```python
from build123d import *

# Parameters (mm, degrees)
FILLET1_R           = 0.2
FILLET2_R           = 1
SKETCH2_R           = 2.5
BOSS_EXTRUDE1_DEPTH = 30
CUT_EXTRUDE1_DEPTH  = 2


with BuildPart() as part:
    # Sketch1 → Revolve1 (revolve)
    with BuildSketch(Plane.XY):
        with BuildLine():
            Line((0, 0), (4.65, 0))
            Line((4.65, 0), (4.65, 1))
            ThreePointArc((4.65, 1), (3.526943142, 2.164793721), (2, 2.7))
            Line((2, 2.7), (0, 2.7))
            Line((0, 2.7), (0, 0))
        make_face()
    revolve(axis=Axis((0, 55, 0), (0, -1, 0)))

    # Fillet1
    fillet1_edges = [part.edges().sort_by_distance(p)[0] for p in [
        (-4.65, 0, 0),
    ]]
    fillet(fillet1_edges, radius=FILLET1_R)

    # Fillet2
    fillet2_edges = [part.edges().sort_by_distance(p)[0] for p in [
        (-4.65, 1, 0),
    ]]
    fillet(fillet2_edges, radius=FILLET2_R)

    # Sketch2 → Boss-Extrude1 (add)
    with BuildSketch(Plane.XZ):
        Circle(SKETCH2_R)
    extrude(amount=BOSS_EXTRUDE1_DEPTH)

    # Sketch6 → Revolve2 (revolve)
    with BuildSketch(Plane.XY):
        Polygon((0, 0), (0, 2.7), (1.274203424, 2.7), (4.45, 0), align=None)
    revolve(axis=Axis((0, 55, 0), (0, -1, 0)))

    # Sketch7 → Cut-Extrude1 (cut)
    with BuildSketch(Plane(origin=(0, 2.7, 0), x_dir=(1, 0, 0), z_dir=(0, 1, 0))):
        Polygon((0.866025404, -1.5), (1.732050808, 0), (0.866025404, 1.5), (-0.866025404, 1.5), (-1.732050808, 0), (-0.866025404, -1.5), align=None)
    extrude(amount=-CUT_EXTRUDE1_DEPTH, mode=Mode.SUBTRACT)

    # Sketch8 → Cut-Revolve1 (revolve, cut)
    with BuildSketch(Plane.XY):
        with BuildLine():
            Line((0, 0.7), (0, 0.2))
            ThreePointArc((0, 0.2), (0.877315732, 0.410889157), (1.732050808, 0.7))
            Line((1.732050808, 0.7), (0, 0.7))
        make_face()
    revolve(axis=Axis((0, 55, 0), (0, -1, 0)), mode=Mode.SUBTRACT)

    # Sketch9 → Cut-Revolve2 (revolve, cut)
    with BuildSketch(Plane.XY):
        with BuildLine():
            ThreePointArc((0, 2.497958971), (1.00508962, 2.548597441), (2, 2.7))
            Line((2, 2.7), (0, 2.7))
            Line((0, 2.7), (0, 2.497958971))
        make_face()
    revolve(axis=Axis((0, 55, 0), (0, -1, 0)), mode=Mode.SUBTRACT)


solid = part.part
```
Model file for the job. Use its own axes, mm. A direction names the side the tool comes from. Give positions to 0.01 mm unless a question says otherwise; leave off trailing zeros. Write each loop counter-clockwise with the first axis right and the second up, starting at its lowest first coordinate (ties: lowest second). Pieces come first, ordered by that corner, then holes. Notation, with made-up numbers: (1.25, 79.5) -> (45.25, 79.5) arc R32 ccw to (45.25, 118.5) -> close; hole circle Ø11 at (60.5, 3). An arc over 180 degrees is marked (long way). Use CSV: the item, a comma, the result in double quotes. Start each with the question number.
1) Cut at A-A on y = -3. List the corners of the cut face in (x, z).
2) Tool access for faces 1 (the flat face through (0, 2, -1.5)), 2 (the cylindrical face through (4.435, 0.454, 1.397)), 3 (the flat face through (-2, 0, -2)): list every direction of +Z, -Z, +X, -X, +Y, -Y with a clear straight run to the whole face (end or side of a thin tool).
3) Two-plate mould, pull along Y, no slides. Class faces 4 (the flat face through (0, -30, 0)), 5 (the flat face through (1.293, 1.688, 0.76)): released by +Y, released by -Y, zero draft, split by the parting line, or undercut.
4) Drill centre lines: L1, parallel to Z at x = -1.5, y = -5; L2, parallel to Y at x = 1.25, z = -3.5. Where is each one in solid material? Low to high.
5) Pin check, flat tips, straight feed: P1, Ø0.9, axis at x = 0, y = 1.5, coming from the +Z side; P2, Ø5, axis at x = -2.5, y = -17.5, coming from the +Z side; P3, Ø2, axis at x = 0.5, z = 0, coming from the +Y side. Stop position of each tip, or through.
Final values:
1,outline,"circle Ø5 at (0, 0)"
2,face 1,"+Y"
2,face 2,"+Y, -Y"
2,face 3,"-Y"
3,face 4,"released by -Y"
3,face 5,"zero draft"
4,L1,"z = -2 to 2"
4,L2,"y = 0 to 2.03"
5,P1,"stops at z = 4.59"
5,P2,"stops at z = 2.5"
5,P3,"stops at y = 0.61"
